Here's how the part is built. I have some questions about the finished solid (model axes, mm). A direction names the side the tool comes from. Give positions to 0.01 mm unless a question says otherwise; leave off trailing zeros. Loops run counter-clockwise (first coordinate to the right, second up) from the corner with the lowest first, then second, coordinate; pieces in that order, holes last. Notation, with made-up numbers: (87, 14) - (106, 14) arc R29 ccw to (106, 42) - close; hole circle Ø10 at (-12.75, 35.25). An arc over 180 degrees is marked (long way). Use one line per item in the form item = value.
from build123d import *

# Parameters (mm, degrees)
SKETCH_1_W                   = 80
SKETCH_1_H                   = 68
EXTRUDE_1_DEPTH              = 10
SKETCH_2_R                   = 19
CUT_EXTRUDE_1_DEPTH          = 10
HOLE_WIZARD_M6_1_D           = 6.6
HOLE_WIZARD_M6_1_CBORE_D     = 11
HOLE_WIZARD_M6_1_CBORE_DEPTH = 4.7
HOLE_WIZARD_M4_1_D           = 3.3
SKETCH_7_R                   = 5
CUT_EXTRUDE_2_DEPTH          = 5


with BuildPart() as part:
    # 草图1 → 凸台-拉伸1 (new body)
    with BuildSketch(Plane.XY):
        with Locations((0, -6)):
            Rectangle(SKETCH_1_W, SKETCH_1_H)
    extrude(amount=-EXTRUDE_1_DEPTH)

    # 草图2 → 切除-拉伸1 (cut)
    with BuildSketch(Plane.XY):
        Circle(SKETCH_2_R)
    extrude(amount=-CUT_EXTRUDE_1_DEPTH, mode=Mode.SUBTRACT)

    # M6 内六角花型圆柱头螺钉的柱形沉头孔1 (through all)
    with Locations(Plane.XY):
        with Locations((30, -30), (-30, -30), (10, -30), (-10, -30)):
            CounterBoreHole(HOLE_WIZARD_M6_1_D / 2, HOLE_WIZARD_M6_1_CBORE_D / 2, HOLE_WIZARD_M6_1_CBORE_DEPTH)

    # M4 螺纹孔1 (through all)
    with Locations(Plane.XY):
        with Locations((23.5, -23.5), (0, 0), (23.5, 23.5), (-23.5, -23.5), (-23.5, 23.5)):
            Hole(HOLE_WIZARD_M4_1_D / 2)

    # 草图7 → 切除-拉伸2 (cut)
    with BuildSketch(Plane.XY.offset(-10)):
        with Locations((30, 0)):
            Circle(SKETCH_7_R)
    cut_extrude_2 = extrude(amount=CUT_EXTRUDE_2_DEPTH, mode=Mode.SUBTRACT)

    # 镜向1: 切除-拉伸2 across plane
    add(cut_extrude_2.mirror(Plane(origin=(0, 0, 0), x_dir=(0, 0, 1), z_dir=(1, 0, 0))), mode=Mode.SUBTRACT)


solid = part.part
(1) Thinking about a two-plate mould opening in X: for faces 1 (the cylindrical face through (8.767, -16.856, -4.93)), 2 (the flat face through (-40, -6, -5)), 3 (the flat face through (-1, -21, -10)), which applies, pulls with the +X half, pulls with the -X half, needs draft (parallel to the pull), parting line crosses it, or undercut?
Geometry says:
face_1 = undercut
face_2 = pulls with the -X half
face_3 = needs draft
(2) For faces 4 (the cylindrical face through (25, 0, -8)), 5 (the cylindrical face through (12.43, -27.77, -7.39)), 6 (the cylindrical face through (-7.043, -25.362, -2.317)), which set-ups out of +Z, -Z, +X, -X, +Y, -Y let a thin tool reach every point of the face, with its end or its side?
Geometry says:
face_4 = -Z
face_5 = +Z, -Z
face_6 = +Z
(3) If we section it at A-A (x = 0): List the corners of the cut face in (y, z) for me, plus the area to 3 significant figures.
Geometry says:
outline = (-40, -10) - (-19, -10) - (-19, 0) - (-40, 0) - close; (19, -10) - (28, -10) - (28, 0) - (19, 0) - close
area = 300 mm²
(4) If we section it at C-C (y = -23.5): List the corners of the cut face in (x, z) for me, plus the area to 3 significant figures.
Geometry says:
outline = (-40, -10) - (-25.15, -10) - (-25.15, 0) - (-40, 0) - close; (-21.85, -10) - (21.85, -10) - (21.85, 0) - (-21.85, 0) - close; (25.15, -10) - (40, -10) - (40, 0) - (25.15, 0) - close
area = 734 mm²
(5) If we section it at B-B (z = -3): Give the number of separate pieces and of enclosed holes in the cut face, plus the area to 3 significant figures.
Geometry says:
separate_pieces = 1
enclosed_holes = 9
area = 3,890 mm²
(6) If I drill on probe 1 along Y at (x, z) = (-23.5, -2.75); probe 2 along Y at (x, z) = (30, -6.1); probe 3 along X at (y, z) = (-33, -2), over which ranges is the centre line in solid material (lowest first)?
Geometry says:
probe_1 = -40 to -25.15, -21.85 to 21.85, 25.15 to 28
probe_2 = -40 to -33.3, -26.7 to -5, 5 to 28
probe_3 = -40 to -34.61, -25.39 to -14.61, -5.39 to 5.39, 14.61 to 25.39, 34.61 to 40
(7) For P1, Ø4, axis at x = -30, y = -30, coming from the -Z side; P2, Ø3.5, axis at x = -12, y = -29.5, coming from the +Z side, each with a flat end and sliding along its axis, tell me the tip position at first contact or that it passes through.
Geometry says:
P1 = through
P2 = -4.7
